from build123d import *

# Parameters (mm, degrees)
F0_W     = 300
F0_H     = 300
F1_DEPTH = 20
F3_DEPTH = 10
F4_DEPTH = 8.8
F6_DEPTH = 1.2


with BuildPart() as f1:
    # F0 (on Top) → F1 (new body)
    with BuildSketch(Plane.XY):
        Rectangle(F0_W, F0_H)
    extrude(amount=F1_DEPTH)

    # F2 (on face) → F3 (cut)
    with BuildSketch(Plane.XY.offset(20)):
        with BuildLine():
            Line((-5, -21.4242852856), (-5, -150))
            Line((-5, -150), (5, -150))
            Line((5, -150), (5, -21.4242852856))
            ThreePointArc((5, -21.4242852856), (0, 22), (-5, -21.4242852856))
        make_face()
    extrude(amount=-F3_DEPTH, mode=Mode.SUBTRACT)

    # F2 (on face) → F4 (cut)
    with BuildSketch(Plane.XY.offset(20)):
        with BuildLine():
            Line((-5, -21.4242852856), (-5, -150))
            Line((-5, -150), (5, -150))
            Line((5, -150), (5, -21.4242852856))
            ThreePointArc((5, -21.4242852856), (0, 22), (-5, -21.4242852856))
        make_face()
    extrude(amount=-F4_DEPTH, mode=Mode.SUBTRACT)

    # F5 (on face) → F6 (join)
    with BuildSketch(Plane.XY.offset(10)):
        with BuildLine():
            ThreePointArc((5, -21.4242852856), (0, -22), (-5, -21.4242852856))
            Line((-5, -21.4242852856), (-5, -150))
            Line((-5, -150), (5, -150))
            Line((5, -150), (5, -21.4242852856))
        make_face()
    extrude(amount=F6_DEPTH)


solid = f1.part
Geometry check sheet. Reference: the model listing, model coordinates, mm. A direction names the side the tool comes from. Give positions to 0.01 mm unless a question says otherwise; leave off trailing zeros. Order: outer loops, then holes, each group sorted by start corner. A loop starts at its lowest first (then second) coordinate and runs counter-clockwise, first axis right, second up.
1) Draft check along Y on faces 3 (the flat face through (-2, 35, 20)), 4 (the flat face through (-2, -150, 10)), 5 (the flat face through (0, 0, 10)), 6 (the flat face through (-2, 150, 10)). Enter one of: released by +Y, released by -Y, zero draft, split by the parting line, or undercut.
Results are:
face 3: zero draft
face 4: released by -Y
face 5: undercut
face 6: released by +Y
2) Material ranges on probe 1 along X at (y, z) = (-120.5, 15.75); probe 2 along X at (y, z) = (0, 14.25); probe 3 along Z at (x, y) = (-3, -20), recorded low to high.
Results are:
probe 1: x = -150 to -5, 5 to 150
probe 2: x = -150 to -22, 22 to 150
probe 3: z = 0 to 10
3) Tool access check on faces 1 (the flat face through (-150, -2, 10)), 2 (the flat face through (-5, -85, 16)). Record the directions out of +Z, -Z, +X, -X, +Y, -Y that give a thin tool (end or side, any length) a straight path to the whole face; none if there is none.
Results are:
face 1: +Z, -Z, -X, +Y, -Y
face 2: +Z, -Y
4) Cross-section at A-A (x = 0). Record the boundary of the cut face in (y, z).
Results are:
outline: (-150, 0) - (150, 0) - (150, 20) - (22, 20) - (22, 10) - (-22, 10) - (-22, 11.2) - (-150, 11.2) - close
5) Cross-section at B-B (y = 0). Record the boundary of the cut face in (x, z), then the cut area to 3 significant figures.
Results are:
outline: (-150, 0) - (150, 0) - (150, 20) - (22, 20) - (22, 10) - (-22, 10) - (-22, 20) - (-150, 20) - close
area: 5,560 mm2
